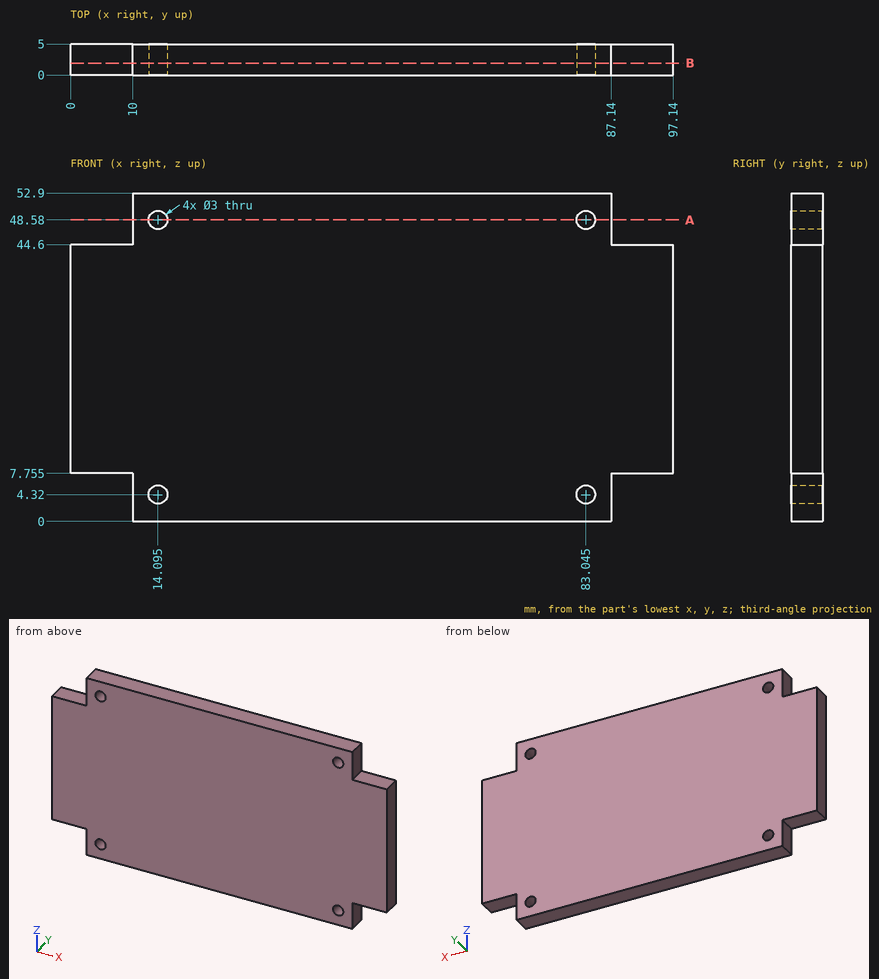
Here's the drawing with two shaded views (mm, measured from the low corner). I have some questions. Coordinates: 2 decimals unless noted, no trailing zeros. Order: outer loops, then holes, each group sorted by start corner. A loop starts at its lowest first (then second) coordinate and runs counter-clockwise, first axis right, second up. Notation, with made-up numbers: (33.5, 11.25) - (79.5, 11.25) arc R8 ccw to (79.5, 22.25) - close; hole circle Ø9 at (13.25, 16.5). An arc over 180 degrees is marked (long way). Use CSV: the item, a comma, the result in double quotes. Start each with the question number.
1. Suppose I cut it at B-B on y = 1.9. List the corners of the cut face in (x, z) for me (1 decimal).
2. Suppose I cut it at A-A on z = 48.58. List the corners of the cut face in (x, y) for me (1 decimal), then the cut area to 3 significant figures.
3. I'm going to push flat-ended pins straight in: pin 1 (1.5 mm diameter, centred on x = 91.5, y = 1.5, fed in from +Z); pin 2 (1.5 mm diameter, centred on y = 1.5, z = 3.5, fed in from +X); pin 3 (2.5 mm diameter, centred on x = 14.095, z = 48.58, fed in from +Y); pin 4 (1.5 mm diameter, centred on y = 3.5, z = 5, fed in from -X). Where does each tip first touch, or does it pass through?
4. Please list where these lines run through material, in increasing order: line 1 (X direction, y = 3.6, z = 4.32) (1 decimal); line 2 (Z direction, x = 83, y = 0.45); line 3 (X direction, y = 0.4, z = 48). Write a range as from..to.
Output:
1,outline,"(0, 7.8) - (10, 7.8) - (10, 0) - (87.1, 0) - (87.1, 7.8) - (97.1, 7.8) - (97.1, 44.6) - (87.1, 44.6) - (87.1, 52.9) - (10, 52.9) - (10, 44.6) - (0, 44.6) - close; hole circle Ø3 at (14.1, 4.3); hole circle Ø3 at (14.1, 48.6); hole circle Ø3 at (83, 4.3); hole circle Ø3 at (83, 48.6)"
2,outline,"(10, 0) - (12.6, 0) - (12.6, 5) - (10, 5) - close; (15.6, 0) - (81.5, 0) - (81.5, 5) - (15.6, 5) - close; (84.5, 0) - (87.1, 0) - (87.1, 5) - (84.5, 5) - close"
2,area,"356 mm2"
3,pin 1,"stops at z = 44.6"
3,pin 2,"stops at x = 87.14"
3,pin 3,"passes through"
3,pin 4,"stops at x = 10"
4,line 1,"x = 10..12.6, 15.6..81.5, 84.5..87.1"
4,line 2,"z = 0..2.82, 5.82..47.08, 50.08..52.9"
4,line 3,"x = 10..12.71, 15.48..81.66, 84.43..87.14"
